Work out the finished part from the listing and answer in its coordinate system (mm). A direction names the side the tool comes from. Coordinates: 2 decimals unless noted, no trailing zeros. Loops run counter-clockwise (first coordinate to the right, second up) from the corner with the lowest first, then second, coordinate; pieces in that order, holes last. Notation, with made-up numbers: (54, -17) - (107, -17) arc R15 cw to (107, -2) - close; hole circle Ø9 at (23.25, 18). An arc over 180 degrees is marked (long way). Write each question's results on one line, items separated by ' | '. Start each with the question number.
1. A cutting plane is placed at A-A on z = 17. Determine the outline of the cut face in (x, y), then the cut area to 3 significant figures.
2. A cutting plane is placed at D-D on z = 2.5. Determine the outline of the cut face in (x, y).
3. Determine the mould class of faces 4 (the flat face through (-29.174, 98, 1)), 5 (the cylindrical face through (-27.83, 74.4, 1.48)), 6 (the flat face through (-13.11, 84.89, 12)) for opening direction X: released by +X, released by -X, zero draft, split by the parting line, or undercut.
4. A cutting plane is placed at C-C on x = -24.5. Determine the outline of the cut face in (y, z).
5. A cutting plane is placed at B-B on y = 104.5. Determine the outline of the cut face in (x, z).
6. Each of these flat-tipped pins is pushed along its axis until it touches: P1, Ø0.6, axis at x = -6, z = 17, coming from the +Y side; P2, Ø2, axis at x = -2.5, z = 10.5, coming from the +Y side; P3, Ø4, axis at y = 97.5, z = 3.5, coming from the +X side; P4, Ø2.5, axis at x = -25.76, y = 88.95, coming from the +Z side. Where does it stop, or does it pass through?
7. Find the intervals of material crossed by line 1 along Z through (x, y) = (11, 85); line 2 along X through (y, z) = (81, 11.25); line 3 along X through (y, z) = (109.5, 9), in increasing order. Write a range as [from, to].
8. Which of the six approach directions +Z, -Z, +X, -X, +Y, -Y give full straight-line access (tool end or side, diameter ignored) to faces 1 (the flat face through (-21.719, 109, 1)), 2 (the flat face through (-12.57, 88.85, 17.01)), 3 (the flat face through (-1, 85, 16))?
from build123d import *

# Parameters (mm, degrees)
SKETCH_1_R       = 2
EXTRUDE_1_DEPTH  = 3
EXTRUDE_2_DEPTH  = 15
SKETCH_3_W       = 2
SKETCH_3_H       = 6
EXTRUDE_3_DEPTH  = 29
SKETCH_5_W       = 2
SKETCH_5_H       = 6
EXTRUDE_4_DEPTH  = 7
SKETCH_6_W       = 32
SKETCH_6_H       = 7
EXTRUDE_5_DEPTH  = 2
CHAMFER_1_SIZE   = 5
SKETCH_8_W       = 32
SKETCH_8_H       = 2.104912686
EXTRUDE_6_DEPTH  = 7
SKETCH_9_W       = 27
SKETCH_9_H       = 4.5
EXTRUDE_7_DEPTH  = 5.5
CHAMFER_2_SIZE   = 5
EXTRUDE_8_DEPTH  = 9.5
CHAMFER_3_SIZE   = 5
CHAMFER_4_SIZE   = 3
CHAMFER_6_SIZE   = 2
CHAMFER_6_SIZE_2 = 11.342563639


with BuildPart() as part:
    # 草图1 → 凸台-拉伸1 (new body)
    with BuildSketch(Plane.XY):
        with BuildLine():
            Line((-22.344972157, 75.303248777), (-15.102670088, 80.384719944))
            Line((-15.102670088, 80.384719944), (-15.102670088, 113.200215401))
            Line((-15.102670088, 113.200215401), (-21.718999147, 113.200215401))
            Line((-21.718999147, 113.200215401), (-21.718999147, 103.843357559))
            ThreePointArc((-21.718999147, 103.843357559), (-22.903426745, 100.983896387), (-25.762887917, 99.799468789))
            Line((-25.762887917, 99.799468789), (-29.17448261, 99.799468789))
            Line((-29.17448261, 99.799468789), (-29.17448261, 97.102223458))
            Line((-29.17448261, 97.102223458), (-30.762887917, 97.102223458))
            Line((-30.762887917, 97.102223458), (-30.762887917, 88.952611989))
            Line((-30.762887917, 88.952611989), (-30.762887917, 78.952611989))
            ThreePointArc((-30.762887917, 78.952611989), (-27.751659045, 74.365151973), (-22.344972157, 75.303248777))
        make_face()
        with Locations((-25.762887917, 88.952611989)):
            Circle(SKETCH_1_R, mode=Mode.SUBTRACT)
        with Locations((-25.762887917, 78.952611989)):
            Circle(SKETCH_1_R, mode=Mode.SUBTRACT)
    extrude(amount=EXTRUDE_1_DEPTH)

    # 草图2 → 凸台-拉伸2 (add)
    with BuildSketch(Plane.XY.offset(3)):
        Polygon((-18.102670088, 80.384719944), (-18.102670088, 78.279807258), (-15.102670088, 80.384719944), (-15.102670088, 113.200215401), (-18.102670088, 113.200215401), align=None)
    extrude(amount=EXTRUDE_2_DEPTH)

    # 草图3 → 凸台-拉伸3 (add)
    with BuildSketch(Plane(origin=(-15.102670088, 0, 0), x_dir=(0, 0, -1), z_dir=(1, 0, 0))):
        with Locations((-17, 83.384719944)):
            Rectangle(SKETCH_3_W, SKETCH_3_H)
    extrude(amount=EXTRUDE_3_DEPTH)

    # 草图5 → 凸台-拉伸4 (add)
    with BuildSketch(Plane(origin=(0, 0, 16), x_dir=(-1, 0, 0), z_dir=(0, 0, -1))):
        with Locations((-12.897329912, 83.384719944)):
            Rectangle(SKETCH_5_W, SKETCH_5_H)
    extrude(amount=EXTRUDE_4_DEPTH)

    # 草图6 → 凸台-拉伸5 (add)
    with BuildSketch(Plane.XY.offset(18)):
        with Locations((-2.102670088, 81.779807258)):
            Rectangle(SKETCH_6_W, SKETCH_6_H)
    extrude(amount=-EXTRUDE_5_DEPTH)

    # 倒角1
    chamfer_1_edges = [part.edges().sort_by_distance(p)[0] for p in [
        (-15.102670088, 86.384719944, 17),
    ]]
    chamfer(chamfer_1_edges, length=CHAMFER_1_SIZE)

    # 草图8 → 凸台-拉伸6 (add)
    with BuildSketch(Plane(origin=(0, 0, 16), x_dir=(-1, 0, 0), z_dir=(0, 0, -1))):
        with Locations((2.102670088, 79.332263601)):
            Rectangle(SKETCH_8_W, SKETCH_8_H)
    extrude(amount=EXTRUDE_6_DEPTH)

    # 草图9 → 凸台-拉伸7 (add)
    with BuildSketch(Plane(origin=(0, 80.384719944, 0), x_dir=(1, 0, 0), z_dir=(0, 1, 0))):
        with Locations((-1.602670088, -11.25)):
            Rectangle(SKETCH_9_W, SKETCH_9_H)
    extrude(amount=EXTRUDE_7_DEPTH)

    # 倒角2
    chamfer_2_edges = [part.edges().sort_by_distance(p)[0] for p in [
        (-15.102670088, 85.884719944, 11.25),
    ]]
    chamfer(chamfer_2_edges, length=CHAMFER_2_SIZE)

    # 草图10 → 凸台-拉伸8 (add)
    with BuildSketch(Plane(origin=(0, 86.384719944, 0), x_dir=(1, 0, 0), z_dir=(0, 1, 0))):
        Polygon((11.897329912, -9), (11.897329912, -16), (10.494123617, -16), (10.494123617, -18), (11.897329912, -18), (13.897329912, -18), (13.897329912, -9), align=None)
    extrude(amount=EXTRUDE_8_DEPTH)

    # 倒角3
    chamfer_3_edges = [part.edges().sort_by_distance(p)[0] for p in [
        (10.494123617, 86.384719944, 17),
    ]]
    chamfer(chamfer_3_edges, length=CHAMFER_3_SIZE)

    # 倒角4
    chamfer_4_edges = [part.edges().sort_by_distance(p)[0] for p in [
        (11.897329912, 85.884719944, 11.25),
    ]]
    chamfer(chamfer_4_edges, length=CHAMFER_4_SIZE)

    # 倒角6
    # the kernel refuses this chamfer: 11.342563639, 2 mm, written as the material it takes off along each edge
    with BuildSketch(Plane(origin=(-35.944000175, 111.726050031, 13.5), x_dir=(0, 0, -1), z_dir=(0.7071067811865472, -0.7071067811865478, 0))) as chamfer_6_piece_1_section:
        Polygon((CHAMFER_6_SIZE, 0), (0, -CHAMFER_6_SIZE_2), (0, 0), align=None)
    chamfer_6_piece_1 = extrude(amount=66.019251147, mode=Mode.PRIVATE)
    chamfer_6_piece_1 = split(chamfer_6_piece_1, bisect_by=Plane(origin=(-15.102670088, 111.726050031, 13.5), z_dir=(1, 0, 0)), keep=Keep.TOP, mode=Mode.PRIVATE)
    chamfer_6_piece_1 = split(chamfer_6_piece_1, bisect_by=Plane(origin=(-35.944000175, 80.384719944, 13.5), z_dir=(0, 1, 0)), keep=Keep.TOP, mode=Mode.PRIVATE)
    chamfer_6_piece_1 = split(chamfer_6_piece_1, bisect_by=Plane(origin=(-35.944000175, 110.604818441, 7.141179669), z_dir=(0, 0.17364817766692733, 0.9848077530122086)), keep=Keep.TOP, mode=Mode.PRIVATE)
    add(chamfer_6_piece_1, mode=Mode.SUBTRACT)
    with BuildSketch(Plane(origin=(-39.576761755, 85.884719944, 13.5), x_dir=(0, 0, -1), z_dir=(1, 0, 0))) as chamfer_6_piece_2_section:
        Polygon((CHAMFER_6_SIZE, 0), (0, -CHAMFER_6_SIZE_2), (0, 0), align=None)
    chamfer_6_piece_2 = extrude(amount=77.948183335, mode=Mode.PRIVATE)
    chamfer_6_piece_2 = split(chamfer_6_piece_2, bisect_by=Plane(origin=(11.897329912, 85.884719944, 13.5), z_dir=(-1, 0, 0)), keep=Keep.TOP, mode=Mode.PRIVATE)
    chamfer_6_piece_2 = split(chamfer_6_piece_2, bisect_by=Plane(origin=(-15.102670088, 85.884719944, 13.5), z_dir=(1, 0, 0)), keep=Keep.TOP, mode=Mode.PRIVATE)
    chamfer_6_piece_2 = split(chamfer_6_piece_2, bisect_by=Plane(origin=(-39.576761755, 80.384719944, 13.5), z_dir=(0, 1, 0)), keep=Keep.TOP, mode=Mode.PRIVATE)
    chamfer_6_piece_2 = split(chamfer_6_piece_2, bisect_by=Plane(origin=(-39.374230212, 86.087251487, 15.124384731), z_dir=(0.12278780396897075, 0.12278780396897053, 0.9848077530122088)), keep=Keep.TOP, mode=Mode.PRIVATE)
    chamfer_6_piece_2 = split(chamfer_6_piece_2, bisect_by=Plane(origin=(-38.604080635, 84.912038824, 5.698704782), z_dir=(-0.12278780396897096, 0.12278780396897111, 0.9848077530122086)), keep=Keep.TOP, mode=Mode.PRIVATE)
    add(chamfer_6_piece_2, mode=Mode.SUBTRACT)
    with BuildSketch(Plane(origin=(32.73866, 109.726050031, 13.5), x_dir=(0.7071067811865475, -0.7071067811865475, 0), z_dir=(-0.7071067811865476, -0.7071067811865476, 0))) as chamfer_6_piece_3_section:
        Polygon((CHAMFER_6_SIZE_2, 0), (0, -CHAMFER_6_SIZE), (0, 0), align=None)
    chamfer_6_piece_3 = extrude(amount=63.190824022, mode=Mode.PRIVATE)
    chamfer_6_piece_3 = split(chamfer_6_piece_3, bisect_by=Plane(origin=(11.897329912, 109.726050031, 13.5), z_dir=(-1, 0, 0)), keep=Keep.TOP, mode=Mode.PRIVATE)
    chamfer_6_piece_3 = split(chamfer_6_piece_3, bisect_by=Plane(origin=(32.73866, 80.384719944, 13.5), z_dir=(0, 1, 0)), keep=Keep.TOP, mode=Mode.PRIVATE)
    chamfer_6_piece_3 = split(chamfer_6_piece_3, bisect_by=Plane(origin=(32.73866, 108.665125821, 7.483199812), z_dir=(0, 0.17364817766692733, 0.9848077530122086)), keep=Keep.TOP, mode=Mode.PRIVATE)
    add(chamfer_6_piece_3, mode=Mode.SUBTRACT)


solid = part.part
Values:
1) outline: (-18.1, 78.28) - (13.9, 78.28) - (13.9, 95.88) - (10.49, 95.88) - (10.49, 91.38) - (5.49, 86.38) - (-10.1, 86.38) - (-15.1, 91.38) - (-15.1, 113.2) - (-18.1, 113.2) - close | area: 397 mm^2
2) outline: (-30.76, 78.95) arc R5 ccw to (-22.34, 75.3) - (-15.1, 80.38) - (-15.1, 113.2) - (-21.72, 113.2) - (-21.72, 103.84) arc R4.04 cw to (-25.76, 99.8) - (-29.17, 99.8) - (-29.17, 97.1) - (-30.76, 97.1) - close; hole circle Ø4 at (-25.76, 78.95); hole circle Ø4 at (-25.76, 88.95)
3) face 4: released by -X | face 5: split by the parting line | face 6: undercut
4) outline: (74.11, 0) - (77.4, 0) - (77.4, 3) - (74.11, 3) - close; (80.5, 0) - (87.4, 0) - (87.4, 3) - (80.5, 3) - close; (90.5, 0) - (100, 0) - (100, 3) - (90.5, 3) - close
5) outline: (-21.72, 0) - (-15.1, 0) - (-15.1, 18) - (-18.1, 18) - (-18.1, 3) - (-21.72, 3) - close
6) P1: y = 86.38 | P2: y = 85.88 | P3: x = -15.1 | P4: through
7) line 1: [9, 11.87], [16, 18] | line 2: [-18.1, 13.9] | line 3: [-18.1, -15.1]
8) face 1: +Z, -Z, -X, +Y | face 2: +Z, -Z, +Y | face 3: +Y
